The listing builds one solid part. Answer for the finished solid, in the listing's coordinates (mm). Give positions to 0.01 mm unless a question says otherwise; leave off trailing zeros. Loops run counter-clockwise (first coordinate to the right, second up) from the corner with the lowest first, then second, coordinate; pieces in that order, holes last.
Item 1: Section B-B, the plane z = 9 is taken. Give the vertices of the cut face in (x, y).
Item 2: Section C-C, the plane x = -1.27 is taken. Give the vertices of the cut face in (y, z).
Item 3: Section D-D, the plane x = -4 is taken. Give the vertices of the cut face in (y, z), and give its area (3 significant figures).
Item 4: Section A-A, the plane y = 0 is taken. Give the vertices of the cut face in (x, z), and give its area (3 significant figures).
Item 5: Consider line 1 along X through (y, z) = (-0.05, 3.25); line 2 along Y through (x, z) = (3.81, 3.25); line 3 along X through (y, z) = (-0.3, 6.25). Determine where each line is inside the solid, lowest interval first.
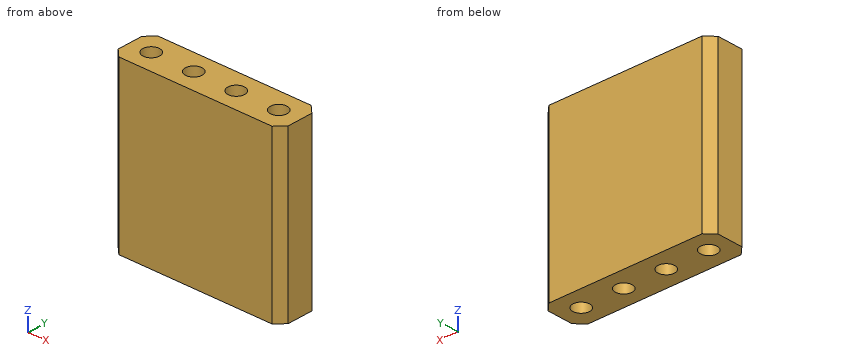
from build123d import *

# Parameters (mm, degrees)
SKETCH_2_W      = 10.16
SKETCH_2_H      = 2.54
SKETCH_2_R      = 0.5
EXTRUDE_1_DEPTH = 10
CHAMFER_2_SIZE  = 0.5


with BuildPart() as part:
    # Эскиз2 → Бобышка-Вытянуть1 (new body)
    with BuildSketch(Plane.XY):
        Rectangle(SKETCH_2_W, SKETCH_2_H)
        with Locations((-3.81, 0)):
            Circle(SKETCH_2_R, mode=Mode.SUBTRACT)
        with Locations((-1.27, 0)):
            Circle(SKETCH_2_R, mode=Mode.SUBTRACT)
        with Locations((1.27, 0)):
            Circle(SKETCH_2_R, mode=Mode.SUBTRACT)
        with Locations((3.81, 0)):
            Circle(SKETCH_2_R, mode=Mode.SUBTRACT)
    extrude(amount=EXTRUDE_1_DEPTH)

    # Фаска2
    chamfer_2_edges = [part.edges().sort_by_distance(p)[0] for p in [
        (5.08, -1.27, 5),
        (-5.08, -1.27, 5),
        (-5.08, 1.27, 5),
        (5.08, 1.27, 5),
    ]]
    chamfer(chamfer_2_edges, length=CHAMFER_2_SIZE)


solid = part.part
Worked answers:
1. outline: (-5.08, -0.77) - (-4.58, -1.27) - (4.58, -1.27) - (5.08, -0.77) - (5.08, 0.77) - (4.58, 1.27) - (-4.58, 1.27) - (-5.08, 0.77) - close; hole circle Ø1 at (-3.81, 0); hole circle Ø1 at (-1.27, 0); hole circle Ø1 at (1.27, 0); hole circle Ø1 at (3.81, 0)
2. outline: (-1.27, 0) - (-0.5, 0) - (-0.5, 10) - (-1.27, 10) - close; (0.5, 0) - (1.27, 0) - (1.27, 10) - (0.5, 10) - close
3. outline: (-1.27, 0) - (-0.46, 0) - (-0.46, 10) - (-1.27, 10) - close; (0.46, 0) - (1.27, 0) - (1.27, 10) - (0.46, 10) - close
3. area: 16.2 mm2
4. outline: (-5.08, 0) - (-4.31, 0) - (-4.31, 10) - (-5.08, 10) - close; (-3.31, 0) - (-1.77, 0) - (-1.77, 10) - (-3.31, 10) - close; (-0.77, 0) - (0.77, 0) - (0.77, 10) - (-0.77, 10) - close; (1.77, 0) - (3.31, 0) - (3.31, 10) - (1.77, 10) - close; (4.31, 0) - (5.08, 0) - (5.08, 10) - (4.31, 10) - close
4. area: 61.6 mm2
5. line 1: x = -5.08 to -4.31, -3.31 to -1.77, -0.77 to 0.77, 1.77 to 3.31, 4.31 to 5.08
5. line 2: y = -1.27 to -0.5, 0.5 to 1.27
5. line 3: x = -5.08 to -4.21, -3.41 to -1.67, -0.87 to 0.87, 1.67 to 3.41, 4.21 to 5.08
